For this review, use the dimensioned drawing (mm, ordinates from the lowest corner) and the shaded views. A direction names the side the tool comes from. Round coordinates to 2 decimals unless told otherwise and drop trailing zeros. Order: outer loops, then holes, each group sorted by start corner. A loop starts at its lowest first (then second) coordinate and runs counter-clockwise, first axis right, second up. Notation, with made-up numbers: (-24, 58.5) - (21, 58.5) arc R20 cw to (21, 86.5) - close; hole circle Ø7 at (50.25, 87.5). An arc over 180 degrees is marked (long way). Write each question's results on one line, items separated by ' | '. Start each with the question number.
(1) For the marked faces 1, 2 and 3, list the 3-axis set-ups (+Z, -Z, +X, -X, +Y, -Y) from which the entire face can be reached by the end or side of a thin tool; tool diameter is ignored.
(2) For L1, parallel to Z at x = 84.5, y = 330; L2, parallel to X at y = 385, z = 99; L3, parallel to X at y = 49, z = 433.5, list the stretches that pass through material, from the lowest coordinate up. Write a range as from..to.
(3) Draft analysis for pull direction Z (two halves, no side actions). For the marked faces 4, 5 and 6, state which applies: pulls with the +Z half, pulls with the -Z half, needs draft (parallel to the pull), parting line crosses it, or undercut.
(4) Insertion check: pin 1 Ø2 at (x, y) = (551, 397.5) entering from -Z; pin 2 Ø5 at (y, z) = (245.5, 347.5) entering from +X; pin 3 Ø12 at (y, z) = (344.5, 400.5) entering from +X; pin 4 Ø1.5 at (x, z) = (492.5, 363) entering from -Y. Each pin has a flat end and moves straight along its axis. Give the tip position at first contact, or say it passes through.
(5) Take a section at D-D, the plane x = 517. Give the boundary of the cut face in (y, z).
(6) Take a section at C-C, the plane z = 120.5. Give the boundary of the cut face in (x, y).
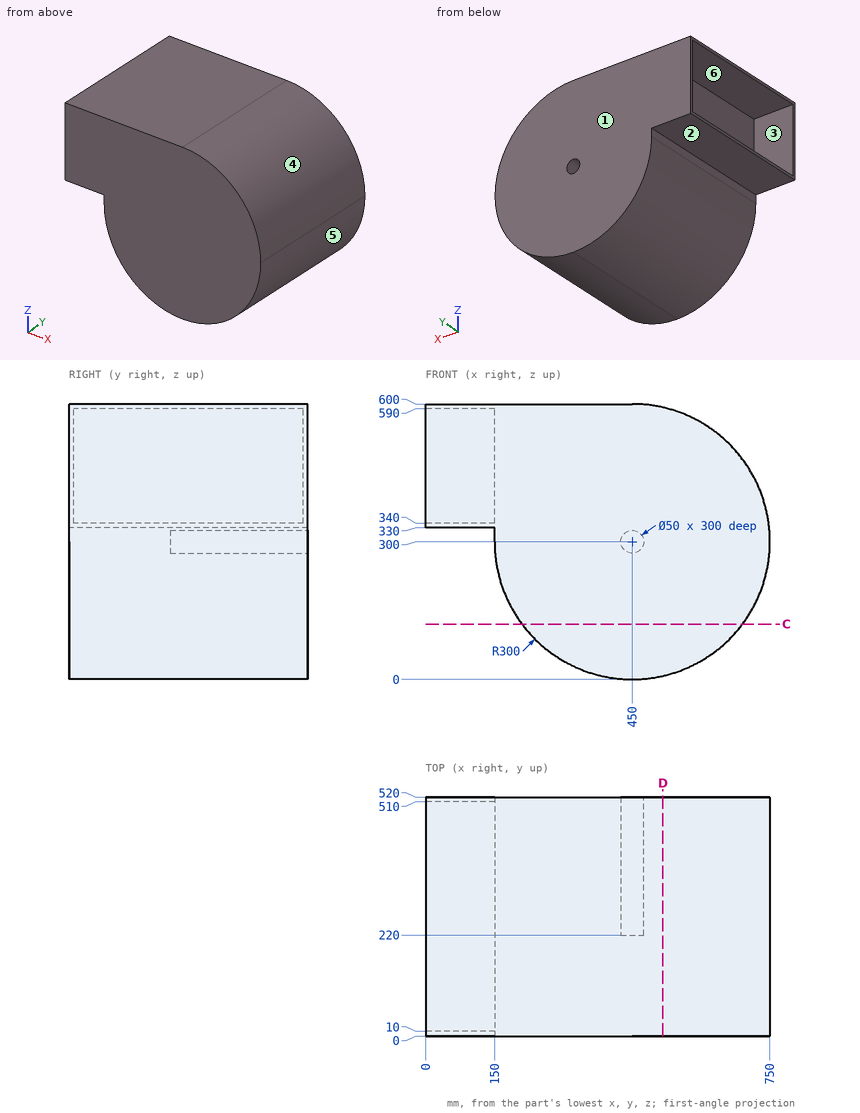
Results below:
1) face 1: +Z, -Z, +X, -X, +Y | face 2: -Z, -X, +Y, -Y | face 3: -X
2) L1: z = 330..340, 590..600 | L2: x = 227.29..672.71 | L3: x = 150..718.66
3) face 4: pulls with the +Z half | face 5: pulls with the -Z half | face 6: undercut
4) pin 1: stops at z = 17.16 | pin 2: stops at x = 746.61 | pin 3: stops at x = 734.73 | pin 4: stops at y = 0
5) outline: (0, 7.58) - (520, 7.58) - (520, 592.42) - (0, 592.42) - close
6) outline: (209.63, 0) - (690.37, 0) - (690.37, 520) - (209.63, 520) - close
